Geometry: final body of the model. Coordinates: model frame, mm. Face numbers are marked on the shaded views. A direction names the side the tool comes from. Give positions to 0.01 mm unless a question says otherwise; leave off trailing zeros. Order: outer loops, then holes, each group sorted by start corner. A loop starts at its lowest first (then second) coordinate and runs counter-clockwise, first axis right, second up. Notation, with made-up numbers: (5, 74) -> (37, 74) arc R19 cw to (37, 96) -> close; hole circle Ø2 at (-7.75, -20). An arc over 180 degrees is marked (long way). One line per question, with ' | ' between items. Start each with the question number.
(1) Ray query, L1, parallel to Y at x = 0, z = 3.35; L2, parallel to Z at x = -15.5, y = 2; L3, parallel to Z at x = 14, y = -22.5. Return the intervals inside material, ascending.
(2) First-contact query: pin 1 Ø0.9 at (x, y) = (13, -6) entering from +Z; pin 2 Ø3 at (x, y) = (13, -6.56) entering from -Z; pin 3 Ø4 at (x, y) = (-3, 22.5) entering from -Z; pin 4 Ø1.5 at (x, z) = (8, 2.5) entering from +Y. Flat tips, straight axial feed; report the tip coordinate or a pass-through.
(3) Section D-D (y = 20). Return loops of the section in (x, z), then the cut area to 3 significant figures.
(4) Section A-A (x = 0). Return loops of the section in (y, z), then the cut area to 3 significant figures.
(5) Set-up query: the marked faces 3 and 4. Return all of +Z, -Z, +X, -X, +Y, -Y with unobstructed straight access to the full face (end or side cutting, diameter ignored); none if empty.
(6) Section C-C (z = 2.3). Return loops of the section in (x, y).
(7) Section B-B (y = 11). Return loops of the section in (x, z), then the cut area to 3 significant figures.
(8) Mould query, pull axis Y, two halves, no side actions, for the marked faces 1 and 2. Classes: +Y half, -Y half, draft (parallel to the pull), parting line (faces both ways), or undercut.
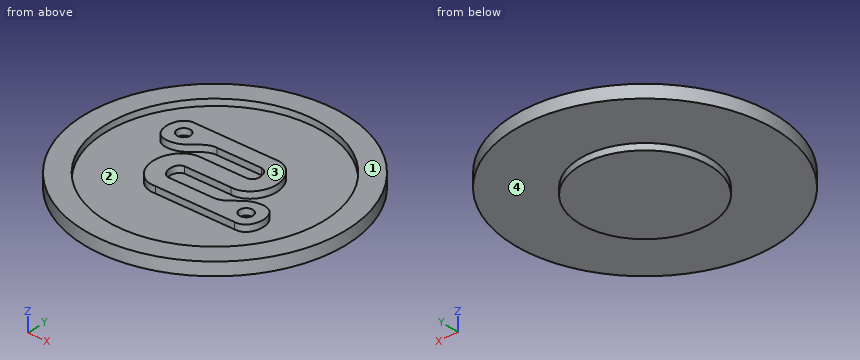
```python
from build123d import *

# Parameters (mm, degrees)
SZKIC2_R                    = 15
DODANIE_WYCI_GNI_CIE1_DEPTH = 1.5
SZKIC3_R                    = 30
DODANIE_WYCI_GNI_CIE2_DEPTH = 1.5
SZKIC4_R                    = 1.549896932
DODANIE_WYCI_GNI_CIE3_DEPTH = 1.5
SZKIC5_R                    = 30
SZKIC5_R_2                  = 25
DODANIE_WYCI_GNI_CIE4_DEPTH = 1.5


with BuildPart() as part:
    # Szkic2 → Dodanie-wyciągnięcie1 (new body)
    with BuildSketch(Plane.XY):
        Circle(SZKIC2_R)
    extrude(amount=DODANIE_WYCI_GNI_CIE1_DEPTH)

    # Szkic3 → Dodanie-wyciągnięcie2 (add)
    with BuildSketch(Plane.XY.offset(1.5)):
        Circle(SZKIC3_R)
    extrude(amount=DODANIE_WYCI_GNI_CIE2_DEPTH)

    # Szkic4 → Dodanie-wyciągnięcie3 (add)
    with BuildSketch(Plane.XY.offset(3)):
        with BuildLine():
            Line((4.812477136, 10.260072193), (-13.590223768, 10.260072193))
            add(Edge.make_bspline(
                [(-13.590223768, 10.260072193), (-17.118745335, 10.525910667), (-18.036890573, 2.046692384), (-9.462596481, 2.827097674), (-7.837333483, 6.548859819), (-5.272128066, 6.55590597)],
                knots=[0, 0, 0, 0, 0.432020753, 0.673133157, 1, 1, 1, 1], degree=3))
            Line((-5.272128066, 6.55590597), (5.077687391, 6.55590597))
            add(Edge.make_bspline(
                [(5.400788266, 2.266678597), (6.693166153, 2.459988983), (7.256310662, 4.478210573), (6.099978239, 6.399808673), (5.077687391, 6.55590597)],
                knots=[0, 0, 0, 0, 0.494793037, 1, 1, 1, 1], degree=3))
            Line((5.400788266, 2.266678597), (-5.393615059, 2.266678597))
            add(Edge.make_bspline(
                [(-4.812477136, -10.260072193), (-8.43662289, -10.67337056), (-13.131808051, -3.70534385), (-8.393582508, 2.373047437), (-5.393615059, 2.266678597)],
                knots=[0, 0, 0, 0, 0.544342745, 1, 1, 1, 1], degree=3))
            Line((-4.812477136, -10.260072193), (13.590223768, -10.260072193))
            add(Edge.make_bspline(
                [(13.590223768, -10.260072193), (17.118745335, -10.525910667), (18.036890573, -2.046692384), (9.462596481, -2.827097674), (7.837333483, -6.548859819), (5.272128066, -6.55590597)],
                knots=[0, 0, 0, 0, 0.432020753, 0.673133157, 1, 1, 1, 1], degree=3))
            Line((5.272128066, -6.55590597), (-5.077687391, -6.55590597))
            add(Edge.make_bspline(
                [(-5.393615059, -1.873220172), (-6.707130139, -2.111629026), (-7.285258718, -4.388625667), (-6.108553028, -6.392911018), (-5.077687391, -6.55590597)],
                knots=[0, 0, 0, 0, 0.526459521, 1, 1, 1, 1], degree=3))
            Line((-5.393615059, -1.873220172), (5.400788266, -1.873220172))
            add(Edge.make_bspline(
                [(4.812477136, 10.260072193), (8.408712031, 10.687954055), (13.196256947, 3.738137397), (8.332970423, -2.090379005), (5.400788266, -1.873220172)],
                knots=[0, 0, 0, 0, 0.552476507, 1, 1, 1, 1], degree=3))
        make_face()
        with Locations((-12.996205696, 6.55590597)):
            Circle(SZKIC4_R, mode=Mode.SUBTRACT)
        with Locations((12.996205696, -6.55590597)):
            Circle(SZKIC4_R, mode=Mode.SUBTRACT)
    extrude(amount=DODANIE_WYCI_GNI_CIE3_DEPTH)

    # Szkic5 → Dodanie-wyciągnięcie4 (add)
    with BuildSketch(Plane.XY.offset(3)):
        Circle(SZKIC5_R)
        Circle(SZKIC5_R_2, mode=Mode.SUBTRACT)
    extrude(amount=DODANIE_WYCI_GNI_CIE4_DEPTH)


solid = part.part
```
Response:
1) L1: y = -30 to -25, -10.26 to -6.56, -1.87 to 2.27, 6.56 to 10.26, 25 to 30 | L2: z = 1.5 to 3 | L3: z = 1.5 to 4.5
2) pin 1: stops at z = 3 | pin 2: stops at z = 0 | pin 3: stops at z = 1.5 | pin 4: stops at y = 29.11
3) outline: (-22.36, 1.5) -> (22.36, 1.5) -> (22.36, 4.5) -> (15, 4.5) -> (15, 3) -> (-15, 3) -> (-15, 4.5) -> (-22.36, 4.5) -> close | area: 89.2 mm^2
4) outline: (-30, 1.5) -> (-15, 1.5) -> (-15, 0) -> (15, 0) -> (15, 1.5) -> (30, 1.5) -> (30, 4.5) -> (25, 4.5) -> (25, 3) -> (10.26, 3) -> (10.26, 4.5) -> (6.56, 4.5) -> (6.56, 3) -> (2.27, 3) -> (2.27, 4.5) -> (-1.87, 4.5) -> (-1.87, 3) -> (-6.56, 3) -> (-6.56, 4.5) -> (-10.26, 4.5) -> (-10.26, 3) -> (-25, 3) -> (-25, 4.5) -> (-30, 4.5) -> close | area: 167 mm^2
5) face 3: +Z, +X, -X, +Y, -Y | face 4: -Z
6) outline: circle Ø60 at (0, 0)
7) outline: (-27.91, 1.5) -> (-10.2, 1.5) -> (-10.2, 0) -> (10.2, 0) -> (10.2, 1.5) -> (27.91, 1.5) -> (27.91, 4.5) -> (22.45, 4.5) -> (22.45, 3) -> (-22.45, 3) -> (-22.45, 4.5) -> (-27.91, 4.5) -> close | area: 131 mm^2
8) face 1: draft | face 2: undercut
